Input: part model. Units: mm. Frame: model coordinates. A direction names the side the tool comes from. Round coordinates to 2 decimals unless told otherwise and drop trailing zeros. Write each loop counter-clockwise with the first axis right and the second up, starting at its lowest first coordinate (ties: lowest second). Pieces come first, ordered by that corner, then holes. Notation, with made-up numbers: (-22, 80.5) -> (26, 80.5) arc R20 ccw to (26, 93.5) -> close; hole circle Ø10 at (70, 34.5). An arc over 180 degrees is marked (long way). Write item = value, one per line.
```python
from build123d import *

# Parameters (mm, degrees)
BOSS_EXTRUDE1_DEPTH = 4


with BuildPart() as part:
    # Layer1 → Boss-Extrude1 (new body)
    with BuildSketch(Plane(origin=(0, 0, 0), x_dir=(1, 0, 0), z_dir=(0, 1, 0))):
        with BuildLine():
            Line((27, 42), (11.25, 42))
            Line((11.25, 42), (11.25, 24))
            Line((11.25, 24), (-11.25, 24))
            Line((-11.25, 24), (-11.25, 42))
            Line((-11.25, 42), (-27, 42))
            ThreePointArc((-27, 42), (-37.606601718, 37.606601718), (-42, 27))
            Line((-42, 27), (-42, 21.5))
            Line((-42, 21.5), (-42, -21.5))
            Line((-42, -21.5), (-42, -27))
            ThreePointArc((-42, -27), (-37.606601718, -37.606601718), (-27, -42))
            Line((-27, -42), (-11.25, -42))
            Line((-11.25, -42), (-11.25, -24))
            Line((-11.25, -24), (11.25, -24))
            Line((11.25, -24), (11.25, -42))
            Line((11.25, -42), (27, -42))
            ThreePointArc((27, -42), (37.606601718, -37.606601718), (42, -27))
            Line((42, -27), (42, 27))
            ThreePointArc((42, 27), (37.606601718, 37.606601718), (27, 42))
        make_face()
    extrude(amount=BOSS_EXTRUDE1_DEPTH)


solid = part.part
```
1) Cut plane C-C (y = 2.7). Return the cut outline in (x, z).
Solutions:
outline = (-42, -27) arc R15 ccw to (-27, -42) -> (-11.25, -42) -> (-11.25, -24) -> (11.25, -24) -> (11.25, -42) -> (27, -42) arc R15 ccw to (42, -27) -> (42, 27) arc R15 ccw to (27, 42) -> (11.25, 42) -> (11.25, 24) -> (-11.25, 24) -> (-11.25, 42) -> (-27, 42) arc R15 ccw to (-42, 27) -> close
2) Draft query along X for faces 4 (the face through (42, 2, 0)), 5 (the face through (-11.25, 2, -33)), 6 (the face through (19, 2, -42)). Return one class per face: +X half, -X half, draft (parallel to the pull), parting line (faces both ways), or undercut.
Solutions:
face_4 = +X half
face_5 = undercut
face_6 = draft
3) Access query for faces 1 (the face through (0, 2, -24)), 2 (the face through (-19, 2, 42)), 3 (the face through (11.25, 2, 33)). Directions: +Z, -Z, +X, -X, +Y, -Y. A direction counts if a zero-diameter tool reaches every point of the face in a straight line with its end or side. Return the directions, or none.
Solutions:
face_1 = -Z, +Y, -Y
face_2 = +Z, +X, -X, +Y, -Y
face_3 = +Z, +Y, -Y
4) Cut plane B-B (z = -36). Return the cut outline in (x, y).
Solutions:
outline = (-39, 0) -> (-11.25, 0) -> (-11.25, 4) -> (-39, 4) -> close; (11.25, 0) -> (39, 0) -> (39, 4) -> (11.25, 4) -> close
5) Cut plane D-D (x = 3). Return the cut outline in (y, z), and give its area (3 significant figures).
Solutions:
outline = (0, -24) -> (4, -24) -> (4, 24) -> (0, 24) -> close
area = 192 mm^2
6) Line query: L1, parallel to X at y = 2.4, z = -27.5; L2, parallel to X at y = 1.75, z = 32; L3, parallel to Z at x = -1, y = 1.9. Output: solid intervals per line, ascending. Write a range as from..to.
Solutions:
L1 = -41.99..-11.25, 11.25..41.99
L2 = -41.14..-11.25, 11.25..41.14
L3 = -24..24
7) Cut plane A-A (z = -26). Return the cut outline in (x, y), and give its area (3 significant figures).
Solutions:
outline = (-42, 0) -> (-11.25, 0) -> (-11.25, 4) -> (-42, 4) -> close; (11.25, 0) -> (42, 0) -> (42, 4) -> (11.25, 4) -> close
area = 246 mm^2
8) First-contact query: P1, Ø3, axis at x = -4, z = -24.5, coming from the -Y side; P2, Ø2, axis at y = 3, z = 32, coming from the +X side; P3, Ø1, axis at y = 2.5, z = 33, coming from the -X side; P4, Ø2, axis at y = 1, z = 29, coming from the +X side. Flat tips, straight axial feed; report the tip coordinate or a pass-through.
Solutions:
P1 = 0
P2 = 41.46
P3 = -40.96
P4 = 41.97
